```python
from build123d import *

# Parameters (mm, degrees)
SKETCH_1_W               = 97
SKETCH_1_H               = 187
EXTRUDE_1_DEPTH          = 3
SKETCH_2_R               = 1.65
CUT_EXTRUDE_1_DEPTH      = 3
SKETCH_3_R               = 4
SKETCH_3_R_2             = 1.65
CUT_EXTRUDE_2_DEPTH      = 3
SKETCH_3_4_R             = 1.65
CUT_EXTRUDE_3_DEPTH      = 3
PATTERN_CIRCULAR_1_COUNT = 4
SKETCH_4_W               = 25
SKETCH_4_H               = 60
EXTRUDE_2_DEPTH          = 3
SKETCH_6_R               = 1.65
CUT_EXTRUDE_5_DEPTH      = 3
CUT_EXTRUDE_8_REACH      = 120.968
SKETCH_9_R               = 6
SKETCH_24_R              = 1.65
CUT_EXTRUDE_15_DEPTH     = 3
SKETCH_33_R              = 1.65
CUT_EXTRUDE_24_DEPTH     = 3
SKETCH_42_R              = 1.65
CUT_EXTRUDE_32_DEPTH     = 3
SKETCH_44_W              = 7
SKETCH_44_H              = 20
CUT_EXTRUDE_34_DEPTH     = 10


with BuildPart() as part:
    # 草图1 → 凸台-拉伸1 (new body)
    with BuildSketch(Plane(origin=(0, 0, 0), x_dir=(1, 0, 0), z_dir=(0, 1, 0))):
        Rectangle(SKETCH_1_W, SKETCH_1_H)
    extrude(amount=EXTRUDE_1_DEPTH)

    # 草图2 → 切除-拉伸1 (cut)
    with BuildSketch(Plane(origin=(0, 3, 0), x_dir=(1, 0, 0), z_dir=(0, 1, 0))):
        with Locations(Location((39.5, -53.5, 0), (0, 0, 270))):
            Circle(SKETCH_2_R)
        with Locations(Location((25.5, -53.5, 0), (0, 0, 270))):
            Circle(SKETCH_2_R)
        with Locations(Location((25.5, -69.5, 0), (0, 0, 90))):
            Circle(SKETCH_2_R)
        with Locations(Location((39.5, -69.5, 0), (0, 0, 90))):
            Circle(SKETCH_2_R)
        with Locations(Location((-39.5, -69.5, 0), (0, 0, 270))):
            Circle(SKETCH_2_R)
        with Locations(Location((-25.5, -69.5, 0), (0, 0, 270))):
            Circle(SKETCH_2_R)
        with Locations(Location((-25.5, -53.5, 0), (0, 0, 90))):
            Circle(SKETCH_2_R)
        with Locations(Location((-39.5, -53.5, 0), (0, 0, 90))):
            Circle(SKETCH_2_R)
        with Locations(Location((-39.5, 53.5, 0), (0, 0, 270))):
            Circle(SKETCH_2_R)
        with Locations(Location((-25.5, 53.5, 0), (0, 0, 270))):
            Circle(SKETCH_2_R)
        with Locations(Location((-25.5, 69.5, 0), (0, 0, 90))):
            Circle(SKETCH_2_R)
        with Locations(Location((-39.5, 69.5, 0), (0, 0, 90))):
            Circle(SKETCH_2_R)
        with Locations(Location((39.5, 69.5, 0), (0, 0, 270))):
            Circle(SKETCH_2_R)
        with Locations(Location((25.5, 69.5, 0), (0, 0, 270))):
            Circle(SKETCH_2_R)
        with Locations(Location((25.5, 53.5, 0), (0, 0, 90))):
            Circle(SKETCH_2_R)
        with Locations(Location((39.5, 53.5, 0), (0, 0, 90))):
            Circle(SKETCH_2_R)
    extrude(amount=-CUT_EXTRUDE_1_DEPTH, mode=Mode.SUBTRACT)

    # 草图3 → 切除-拉伸2 (cut)
    with BuildSketch(Plane(origin=(0, 3, 0), x_dir=(1, 0, 0), z_dir=(0, 1, 0))):
        with Locations(Location((0, -22.5, 0), (0, 0, 270))):
            Circle(SKETCH_3_R)
        with Locations(Location((-18.5, -22.5, 0), (0, 0, 270))):
            Circle(SKETCH_3_R_2)
        with Locations(Location((18.5, -22.5, 0), (0, 0, 90))):
            Circle(SKETCH_3_R_2)
    extrude(amount=-CUT_EXTRUDE_2_DEPTH, mode=Mode.SUBTRACT)

    # 草图3<4> → 切除-拉伸3 (cut)
    with BuildSketch(Plane(origin=(0, 3, 0), x_dir=(1, 0, 0), z_dir=(0, 1, 0))):
        with Locations(Location((-7, -22.5, 0), (0, 0, 270))):
            Circle(SKETCH_3_4_R)
    cut_extrude_3 = extrude(amount=-CUT_EXTRUDE_3_DEPTH, mode=Mode.SUBTRACT)

    # 阵列(圆周)1: 切除-拉伸3 ×4 about axis
    pattern_circular_1_axis = Axis((0, 0, 22.5), (0, 1, 0))
    for i in range(1, PATTERN_CIRCULAR_1_COUNT):
        add(cut_extrude_3.rotate(pattern_circular_1_axis, i * 360 / PATTERN_CIRCULAR_1_COUNT), mode=Mode.SUBTRACT)

    # 草图4 → 凸台-拉伸2 (add)
    with BuildSketch(Plane(origin=(0, 3, 0), x_dir=(1, 0, 0), z_dir=(0, 1, 0))):
        with Locations((61, 0)):
            Rectangle(SKETCH_4_W, SKETCH_4_H)
    extrude_2 = extrude(amount=-EXTRUDE_2_DEPTH)

    # 镜向1: 凸台-拉伸2 across plane
    add(extrude_2.mirror(Plane(origin=(0, 0, 0), x_dir=(0, 0, 1), z_dir=(1, 0, 0))))

    # 草图6 → 切除-拉伸5 (cut)
    with BuildSketch(Plane.XZ):
        with Locations(Location((-5, 90.5, 0), (0, 0, 270))):
            Circle(SKETCH_6_R)
        with Locations(Location((15, 90.5, 0), (0, 0, 270))):
            Circle(SKETCH_6_R)
        with Locations(Location((-5, -90.5, 0), (0, 0, 270))):
            Circle(SKETCH_6_R)
        with Locations(Location((15, -90.5, 0), (0, 0, 270))):
            Circle(SKETCH_6_R)
    extrude(amount=-CUT_EXTRUDE_5_DEPTH, mode=Mode.SUBTRACT)

    # 草图9 → 切除-拉伸8 (cut, up to next)
    with BuildSketch(Plane(origin=(0, 3, 0), x_dir=(1, 0, 0), z_dir=(0, 1, 0)), mode=Mode.PRIVATE) as cut_extrude_8_sk1:
        with Locations(Location((-18, -22.5, 0), (0, 0, 270))):
            Circle(SKETCH_9_R)
    cut_extrude_8_tool1 = extrude(cut_extrude_8_sk1.sketch, amount=-CUT_EXTRUDE_8_REACH, mode=Mode.PRIVATE) & part.part
    # 草图9 → 切除-拉伸8 (cut, up to next)
    with BuildSketch(Plane(origin=(0, 3, 0), x_dir=(1, 0, 0), z_dir=(0, 1, 0)), mode=Mode.PRIVATE) as cut_extrude_8_sk2:
        with Locations(Location((18, -22.5, 0), (0, 0, 270))):
            Circle(SKETCH_9_R)
    cut_extrude_8_tool2 = extrude(cut_extrude_8_sk2.sketch, amount=-CUT_EXTRUDE_8_REACH, mode=Mode.PRIVATE) & part.part
    add(cut_extrude_8_tool1.solids().sort_by_distance((-18, 3, 22.5))[0], mode=Mode.SUBTRACT)
    add(cut_extrude_8_tool2.solids().sort_by_distance((18, 3, 22.5))[0], mode=Mode.SUBTRACT)

    # 草图24 → 切除-拉伸15 (cut)
    with BuildSketch(Plane(origin=(0, 3, 0), x_dir=(1, 0, 0), z_dir=(0, 1, 0))):
        with Locations(Location((-22.5, -78.5, 0), (0, 0, 270))):
            Circle(SKETCH_24_R)
        with Locations(Location((22.5, -78.5, 0), (0, 0, 270))):
            Circle(SKETCH_24_R)
        with Locations(Location((22.5, 78.5, 0), (0, 0, 270))):
            Circle(SKETCH_24_R)
        with Locations(Location((-22.5, 78.5, 0), (0, 0, 270))):
            Circle(SKETCH_24_R)
        with Locations((-100.151505846, -27.458044015)):
            Circle(SKETCH_24_R)
        with Locations((-95.406327774, 17.291070893)):
            Circle(SKETCH_24_R)
        with Locations(Location((58.5, -22.5, 0), (0, 0, 270))):
            Circle(SKETCH_24_R)
        with Locations(Location((58.5, 22.5, 0), (0, 0, 270))):
            Circle(SKETCH_24_R)
    extrude(amount=-CUT_EXTRUDE_15_DEPTH, mode=Mode.SUBTRACT)

    # 草图33 → 切除-拉伸24 (cut)
    with BuildSketch(Plane.XZ):
        with Locations(Location((70.5, -5, 0), (0, 0, 270))):
            Circle(SKETCH_33_R)
        with Locations(Location((70.5, 15, 0), (0, 0, 270))):
            Circle(SKETCH_33_R)
        with Locations(Location((-70.5, -5, 0), (0, 0, 270))):
            Circle(SKETCH_33_R)
        with Locations(Location((-70.5, 15, 0), (0, 0, 270))):
            Circle(SKETCH_33_R)
    extrude(amount=-CUT_EXTRUDE_24_DEPTH, mode=Mode.SUBTRACT)

    # 草图42 → 切除-拉伸32 (cut)
    with BuildSketch(Plane(origin=(0, 3, 0), x_dir=(1, 0, 0), z_dir=(0, 1, 0))):
        with Locations(Location((-58.5, 22.5, 0), (0, 0, 270))):
            Circle(SKETCH_42_R)
        with Locations(Location((-58.5, -22.5, 0), (0, 0, 270))):
            Circle(SKETCH_42_R)
    extrude(amount=-CUT_EXTRUDE_32_DEPTH, mode=Mode.SUBTRACT)

    # 草图44 → 切除-拉伸34 (cut)
    with BuildSketch(Plane(origin=(0, 3, 0), x_dir=(1, 0, 0), z_dir=(0, 1, 0))):
        with Locations((-47, 10)):
            Rectangle(SKETCH_44_W, SKETCH_44_H)
        with Locations((47, 10)):
            Rectangle(SKETCH_44_W, SKETCH_44_H)
    extrude(amount=-CUT_EXTRUDE_34_DEPTH, mode=Mode.SUBTRACT)


solid = part.part
```
Verification items for the finished model (mm, model axes). Give positions to 0.01 mm unless a question says otherwise; leave off trailing zeros. Order: outer loops, then holes, each group sorted by start corner. A loop starts at its lowest first (then second) coordinate and runs counter-clockwise, first axis right, second up. Notation, with made-up numbers: M 31,65 L 36,65 A14 ccw 36,72 Z; hole C 13,6 d7. An arc over 180 degrees is marked long. Answer in a Markdown table with one row per item. Add a question column.
Item 1: Section check B-B, the plane y = 0.7. State how many separate pieces and enclosed holes the cut face has, and give its area (3 significant figures).
Item 2: Gauge pin test, flat end, axial feed: pin 1 (1.5 mm diameter, centred on y = 1, z = 47, fed in from -X). Record the tip position at first contact, or that the pin passes through.
Item 3: Section check A-A, the plane x = 54. Enter the section's corners in (y, z), and give its area (3 significant figures).
Item 4: Mould release check, pull along X, two halves, no side actions. Record for faces 1 (the cylindrical face through (-13.94, 1.52, 18.08)), 2 (the flat face through (-1, 0, -1)): released by +X, released by -X, zero draft, split by the parting line, or undercut.
Item 5: Scan lines: probe 1 along X at (y, z) = (1.1, -90.5); probe 2 along X at (y, z) = (1.2, 53.5); probe 3 along X at (y, z) = (2.4, -0.5). Record each from-to range of solid material in increasing order. Write a range as from..to.
Filled sheet:
| question | item | result |
|---|---|---|
| 1 | separate pieces | 1 |
| 1 | enclosed holes | 41 |
| 1 | area | 20,300 mm^2 |
| 2 | pin 1 | stops at x = -48.5 |
| 3 | outline | M 0,-30 L 3,-30 L 3,30 L 0,30 Z |
| 3 | area | 180 mm^2 |
| 4 | face 1 | undercut |
| 4 | face 2 | zero draft |
| 5 | probe 1 | x = -48.5..-6.65, -3.35..13.35, 16.65..48.5 |
| 5 | probe 2 | x = -48.5..-41.15, -37.85..-27.15, -23.85..23.85, 27.15..37.85, 41.15..48.5 |
| 5 | probe 3 | x = -73.5..-50.5, -43.5..43.5, 50.5..73.5 |
